Source: CAD feature listing. Evaluate the final solid. Frame: model axes, mm. Face numbers are marked on the shaded views. A direction names the side the tool comes from. Coordinates: 2 decimals unless noted, no trailing zeros. Write each loop counter-clockwise with the first axis right and the second up, starting at its lowest first coordinate (ties: lowest second). Pieces come first, ordered by that corner, then holes. Notation, with made-up numbers: (-7, -23) -> (35, -23) arc R14 ccw to (35, -4) -> close; hole circle Ø4 at (66.25, 28). An arc over 180 degrees is marked (long way). One line per item, written item: value. Start each with the question number.
1. Access query for the marked faces 1, 2, 3 and 4. Directions: +Z, -Z, +X, -X, +Y, -Y. A direction counts if a zero-diameter tool reaches every point of the face in a straight line with its end or side. Return the directions, or none.
2. Section query C-C, the plane y = -40.5. Output: boundary loops of the cut face in (x, z).
3. Section query D-D, the plane z = 14. Output: boundary loops of the cut face in (x, y) (3 decimals).
4. First-contact query: P1, Ø20, axis at y = -29, z = 16, coming from the +X side; P2, Ø8, axis at y = -0.5, z = -10, coming from the -X side; P3, Ø14.5, axis at y = -25.48, z = 17.73, coming from the -X side; P4, Ø10, axis at x = -22.5, y = -33.5, coming from the -Z side. Flat tips, straight axial feed; report the tip coordinate or a pass-through.
5. Section query B-B, the plane z = 1. Output: boundary loops of the cut face in (x, y).
6. Line query: line 1 (Y direction, x = 36, z = -15); line 2 (Z direction, x = -7, y = -11); line 3 (X direction, y = -25.5, z = 25). Output: solid intervals per line, ascending.
7. Section query A-A, the plane x = -23. Output: boundary loops of the cut face in (y, z), and give its area (3 significant figures).
from build123d import *

# Parameters (mm, degrees)
F2_DEPTH = 50.8
F3_DEPTH = 12.7
F4_R     = 9.161038
F5_DEPTH = 50.8


with BuildPart() as f2:
    # F0 (on Front) → F2 (new body)
    with BuildSketch(Plane.XZ):
        Polygon((-45.646802, -32.811075), (45.646802, -32.811075), (0, 32.811075), (-45.646802, 32.811075), align=None)
    extrude(amount=F2_DEPTH)

    # F1 (on Front) → F3 (join)
    with BuildSketch(Plane.XZ):
        Polygon((4.530817, 37.287548), (-50.311431, 37.287548), (-50.311431, -37.287548), (50.311431, -37.287548), (56.298688, -37.287548), (50.311431, -30.283526), align=None)
    extrude(amount=-F3_DEPTH)

    # F4 (on Right) → F5 (cut)
    with BuildSketch(Plane.YZ):
        with Locations((-25.475649, 17.725538)):
            Circle(F4_R)
    extrude(amount=F5_DEPTH, mode=Mode.SUBTRACT)


solid = f2.part
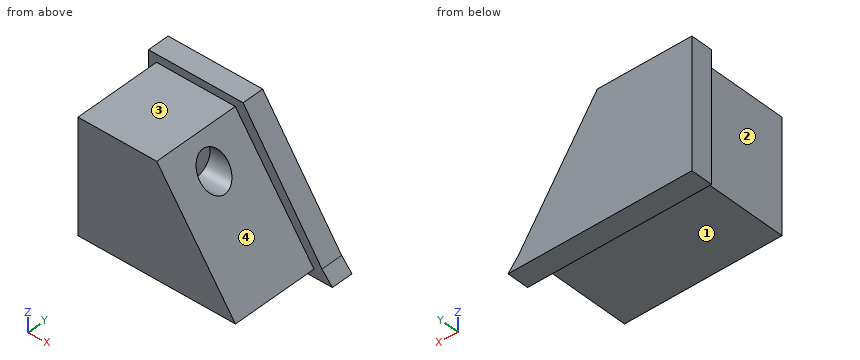
Computed values:
1. face 1: -Z, +X, -X, -Y
1. face 2: +Z, -Z, -X, -Y
1. face 3: +Z, +X, -X, -Y
1. face 4: +Z, +X, -Y
2. outline: (-45.65, -32.81) -> (45.65, -32.81) -> (0, 32.81) -> (-45.65, 32.81) -> close
3. outline: (-50.311, 0) -> (-45.647, 0) -> (-45.647, -50.8) -> (13.085, -50.8) -> (13.085, -33.845) -> (0, -33.845) -> (0, -17.106) -> (13.085, -17.106) -> (13.085, 0) -> (20.309, 0) -> (20.309, 12.7) -> (-50.311, 12.7) -> close
4. P1: stops at x = 18.65
4. P2: stops at x = -50.31
4. P3: stops at x = -45.65
4. P4: stops at z = -32.81
5. outline: (-50.31, 0) -> (-45.65, 0) -> (-45.65, -50.8) -> (22.13, -50.8) -> (22.13, 0) -> (29.12, 0) -> (29.12, 12.7) -> (-50.31, 12.7) -> close
6. line 1: y = 0 to 12.7
6. line 2: z = -32.81 to 32.81
6. line 3: x = -45.65 to 0
7. outline: (-50.8, -32.81) -> (0, -32.81) -> (0, -37.29) -> (12.7, -37.29) -> (12.7, 37.29) -> (0, 37.29) -> (0, 32.81) -> (-50.8, 32.81) -> close
7. area: 4,280 mm²
